```python
from build123d import *

# Parameters (mm, degrees)
BOSS_EXTRUDE1_DEPTH = 14.45
SKETCH2_R           = 1.651
CUT_EXTRUDE1_DEPTH  = 6.35


with BuildPart() as part:
    # Sketch1 → Boss-Extrude1 (new, symmetric)
    with BuildSketch(Plane(origin=(0, 0, 0), x_dir=(0, 0, -1), z_dir=(1, 0, 0))):
        Polygon((0, 0), (10, 0), (10, -8), (4.5, -8), (4.5, -3.5), (-4.5, -3.5), (-4.5, -8), (-10, -8), (-10, 0), align=None)
    extrude(amount=BOSS_EXTRUDE1_DEPTH, both=True)

    # Sketch2 → Cut-Extrude1 (cut)
    with BuildSketch(Plane(origin=(0, 0, 0), x_dir=(1, 0, 0), z_dir=(0, 1, 0))):
        with Locations(Location((5, 7.5, 0), (0, 0, 270))):
            Circle(SKETCH2_R)
        with Locations(Location((5, -7.5, 0), (0, 0, 270))):
            Circle(SKETCH2_R)
        with Locations(Location((-5, -7.5, 0), (0, 0, 270))):
            Circle(SKETCH2_R)
        with Locations(Location((-5, 7.5, 0), (0, 0, 270))):
            Circle(SKETCH2_R)
    extrude(amount=-CUT_EXTRUDE1_DEPTH, mode=Mode.SUBTRACT)


solid = part.part
```
Geometry: final body of the model. Coordinates: model frame, mm. A direction names the side the tool comes from. Coordinates: 2 decimals unless noted, no trailing zeros. Order: outer loops, then holes, each group sorted by start corner. A loop starts at its lowest first (then second) coordinate and runs counter-clockwise, first axis right, second up. Notation, with made-up numbers: (3.25, 81.5) - (51.25, 81.5) arc R33 ccw to (51.25, 109.5) - close; hole circle Ø1 at (-9, 55.5). An arc over 180 degrees is marked (long way). Return JSON: item names as keys, results as strings. Group by question number.
1. Pull-direction query (Z, two-part tool) for faces 4 (the face through (0, -4, 10)), 5 (the face through (0, 0, 0)), 6 (the face through (-5, -6.35, 7)), 7 (the face through (0, -6, -4.5)); classes: pulls with the +Z half, pulls with the -Z half, needs draft (parallel to the pull), parting line crosses it, or undercut.
2. Cut plane C-C (y = -7.5). Output: boundary loops of the cut face in (x, z), plus the area to 3 significant figures.
3. Pin query (flat end, axial travel): pin 1 (7 mm diameter, centred on x = -6.5, z = -0.5, fed in from -Y); pin 2 (1 mm diameter, centred on x = -5.5, z = -8, fed in from +Y). Return the tip coordinate at first contact, or that it passes through.
4. Set-up query: faces 1 (the face through (0, -8, -7)), 2 (the face through (0, -6, 4.5)), 3 (the face through (-4.93, -3.13, 5.85)). Return all of +Z, -Z, +X, -X, +Y, -Y with unobstructed straight access to the full face (end or side cutting, diameter ignored); none if empty.
5. Cut plane D-D (x = -5). Output: boundary loops of the cut face in (y, z).
6. Cut plane A-A (y = -5). Output: boundary loops of the cut face in (x, z), plus the area to 3 significant figures.
7. Cut plane B-B (y = -0.75). Output: boundary loops of the cut face in (x, z).
8. Material intervals for line 1 along X through (y, z) = (-2.75, -7.5); line 2 along X through (y, z) = (-3.5, -7.25); line 3 along Z through (x, y) = (-3, -3.75), sorted ascending. Write a range as [from, to].
Resolved:
{
 "1": {"face 4": "pulls with the +Z half", "face 5": "needs draft", "face 6": "undercut", "face 7": "undercut"},
 "2": {"outline": "(-14.45, -10) - (14.45, -10) - (14.45, -4.5) - (-14.45, -4.5) - close; (-14.45, 4.5) - (14.45, 4.5) - (14.45, 10) - (-14.45, 10) - close", "area": "318 mm²"},
 "3": {"pin 1": "stops at y = -3.5", "pin 2": "stops at y = -6.35"},
 "4": {"face 1": "+Z, -Z, +X, -X, -Y", "face 2": "+X, -X, -Y", "face 3": "+Y"},
 "5": {"outline": "(-8, -10) - (0, -10) - (0, -9.15) - (-6.35, -9.15) - (-6.35, -5.85) - (0, -5.85) - (0, 5.85) - (-6.35, 5.85) - (-6.35, 9.15) - (0, 9.15) - (0, 10) - (-8, 10) - (-8, 4.5) - (-3.5, 4.5) - (-3.5, -4.5) - (-8, -4.5) - close"},
 "6": {"outline": "(-14.45, -10) - (14.45, -10) - (14.45, -4.5) - (-14.45, -4.5) - close; (-14.45, 4.5) - (14.45, 4.5) - (14.45, 10) - (-14.45, 10) - close; hole circle Ø3.3 at (-5, -7.5); hole circle Ø3.3 at (-5, 7.5); hole circle Ø3.3 at (5, -7.5); hole circle Ø3.3 at (5, 7.5)", "area": "284 mm²"},
 "7": {"outline": "(-14.45, -10) - (14.45, -10) - (14.45, 10) - (-14.45, 10) - close; hole circle Ø3.3 at (-5, -7.5); hole circle Ø3.3 at (-5, 7.5); hole circle Ø3.3 at (5, -7.5); hole circle Ø3.3 at (5, 7.5)"},
 "8": {"line 1": "x = [-14.45, -6.65], [-3.35, 3.35], [6.65, 14.45]", "line 2": "x = [-14.45, -6.63], [-3.37, 3.37], [6.63, 14.45]", "line 3": "z = [-10, -4.5], [4.5, 10]"}
}
